Geometry: final body of the model. Coordinates: model frame, mm. A direction names the side the tool comes from. Round coordinates to 2 decimals unless told otherwise and drop trailing zeros. Order: outer loops, then holes, each group sorted by start corner. A loop starts at its lowest first (then second) coordinate and runs counter-clockwise, first axis right, second up. Notation, with made-up numbers: (64.25, 32.5) -> (119.25, 32.5) arc R24 ccw to (119.25, 68.5) -> close; hole circle Ø2 at (-37.75, 11.25). An arc over 180 degrees is marked (long way). Put each result on its own line as item: value.
Autodesk Inventor part; units mm, degrees
ref_plane "YZ Plane" through (0, 0, 0) normal (1, 0, 0) x (0, 1, 0)
ref_plane "XZ Plane" through (0, 0, 0) normal (0, 1, 0) x (-1, 0, 0)
ref_plane "XY Plane" through (0, 0, 0) normal (0, 0, 1) x (1, 0, 0)
sketch "Sketch1" plane through (0, 0, 0) normal (0, 1, 0) x (-1, 0, 0)
  line L0 (-10, 16.5) -> (10, 16.5)
  line L1 (10, 16.5) -> (10, -16.5)
  line L2 (10, -16.5) -> (-10, -16.5)
  line L3 (-10, -16.5) -> (-10, 16.5)
  line L4 (-10, 16.5) -> (10, -16.5) construction
  line L5 (10, 16.5) -> (-10, -16.5) construction
  point P0 (0, 0)
  dimension "d0" = 20
  dimension "d1" = 33
extrude "Extrusion1" add sketch "Sketch1" along normal blind 26
sketch "Sketch2" plane through (10, 0, 16.5) normal (1, 0, 0) x (0, 0, -1)
  line L0 (0, 26) -> (33, 26)
  line L1 (0, 26) -> (0, 21)
  line L2 (0, 0) -> (0, 26)
  line L3 (10, 21) -> (28, 21)
  line L4 (33, 0) -> (33, 26)
  line L5 (33, 26) -> (28, 26)
  line L6 (28, 21) -> (28, 5)
  line L7 (33, 0) -> (0, 0)
  line L8 (33, 0) -> (33, 5)
  line L9 (28, 5) -> (10, 5)
  line L10 (0, 26) -> (10, 26)
  line L11 (10, 21) -> (10, 5)
  point P0 (16.5, 0)
  dimension "d4" = 5
  dimension "d5" = 5
  dimension "d6" = 5
  dimension "d7" = 10
extrude "Extrusion2" cut sketch "Sketch2" against normal blind 26 contours L3 L6 L9 L11
properties part number "Syring Mount"
1. Contact query for a flat-ended pin moving along its axis: P1, Ø12, axis at y = 9.5, z = 4.5, coming from the -X side. Output: stop coordinate, or through.
Ans:
P1: x = -10
2. Cut plane C-C on x = -3.5. Return loops of the section in (y, z).
Ans:
outline: (0, -16.5) -> (26, -16.5) -> (26, 16.5) -> (0, 16.5) -> close; hole (5, -11.5) -> (21, -11.5) -> (21, 6.5) -> (5, 6.5) -> close
3. Cut plane B-B on z = -6.5. Return loops of the section in (x, y), and give its area (3 significant figures).
Ans:
outline: (-10, 0) -> (10, 0) -> (10, 5) -> (-10, 5) -> close; (-10, 21) -> (10, 21) -> (10, 26) -> (-10, 26) -> close
area: 200 mm²
4. Material intervals for probe 1 along Y at (x, z) = (-8, 2); probe 2 along Z at (x, y) = (5.25, 19.5), sorted ascending.
Ans:
probe 1: 0 to 5, 21 to 26
probe 2: -16.5 to -11.5, 6.5 to 16.5
5. Set-up query: faces 1 (the face through (10, 13, 7)), 2 (the face through (0, 21, -2)). Return all of +Z, -Z, +X, -X, +Y, -Y with unobstructed straight access to the full face (end or side cutting, diameter ignored); none if empty.
Ans:
face 1: +Z, -Z, +X, +Y, -Y
face 2: +X, -X
6. Cut plane A-A on y = 17.5. Return loops of the section in (x, z).
Ans:
outline: (-10, -16.5) -> (10, -16.5) -> (10, -11.5) -> (-10, -11.5) -> close; (-10, 6.5) -> (10, 6.5) -> (10, 16.5) -> (-10, 16.5) -> close
7. Draft query along Z for faces 3 (the face through (0, 13, -16.5)), 4 (the face through (0, 13, -11.5)), 5 (the face through (0, 0, 0)). Return one class per face: +Z half, -Z half, draft (parallel to the pull), parting line (faces both ways), or undercut.
Ans:
face 3: -Z half
face 4: undercut
face 5: draft
